```python
from build123d import *

# Parameters (mm, degrees)
CHAMFER_1_SIZE = 3


with BuildPart() as part:
    # Эскиз1 → Повернуть1 (revolve)
    with BuildSketch(Plane.XY):
        Polygon((9, 0), (20, 0), (20, 3.5), (15, 3.5), (15, 8), (12, 36), (5.5, 36), (5.5, 33), (9, 33), align=None)
    revolve(axis=Axis((0, 0, 0), (0, 1, 0)))

    # Эскиз2 → Вырез-Повернуть1 (revolve, cut)
    with BuildSketch(Plane.XY):
        with BuildLine():
            Line((13.5, -3.5), (13.5, -0.5))
            ThreePointArc((13.5, -0.5), (15.5, 1.5), (17.5, -0.5))
            Line((17.5, -0.5), (17.5, -3.5))
            ThreePointArc((17.5, -3.5), (15.5, -5.5), (13.5, -3.5))
        make_face()
    revolve(axis=Axis((0, 0, 0), (0, 1, 0)), mode=Mode.SUBTRACT)

    # Фаска1
    chamfer_1_edges = [part.edges().sort_by_distance(p)[0] for p in [
        (-9, 0, 0),
    ]]
    chamfer(chamfer_1_edges, length=CHAMFER_1_SIZE)


solid = part.part
```
Geometry: final body of the model. Coordinates: model frame, mm. A direction names the side the tool comes from. Coordinates: 2 decimals unless noted, no trailing zeros. Order: outer loops, then holes, each group sorted by start corner. A loop starts at its lowest first (then second) coordinate and runs counter-clockwise, first axis right, second up.
Item 1: Contact query for flat-ended pins moving along their axis: P1, Ø14.5, axis at x = 0, z = 0, coming from the +Y side; P2, Ø14.5, axis at x = 2.5, z = -2.5, coming from the -Y side; P3, Ø1.5, axis at x = -6, y = 6, coming from the -Z side; P4, Ø3, axis at x = 12.5, y = 17, coming from the +Z side. Output: stop coordinate, or through.
Answer:
P1: stops at y = 36
P2: stops at y = 1.21
P3: stops at z = -14.05
P4: stops at z = 8.74
Item 2: Section query B-B (x = 0). Output: boundary loops of the cut face in (y, z).
Answer:
outline: (0, -20) - (3.5, -20) - (3.5, -15) - (8, -15) - (36, -12) - (36, -5.5) - (33, -5.5) - (33, -9) - (3, -9) - (0, -12) - (0, -13.56) arc R2 cw to (0, -17.44) - close; (0, 12) - (3, 9) - (33, 9) - (33, 5.5) - (36, 5.5) - (36, 12) - (8, 15) - (3.5, 15) - (3.5, 20) - (0, 20) - (0, 17.44) arc R2 cw to (0, 13.56) - close
Item 3: Material intervals for line 1 along Y through (x, z) = (17, 9.5); line 2 along Z through (x, y) = (6, 14); line 3 along X through (y, z) = (22.5, 0), sorted ascending.
Answer:
line 1: y = 0 to 3.5
line 2: z = -13.04 to -6.71, 6.71 to 13.04
line 3: x = -13.45 to -9, 9 to 13.45
Item 4: Section query C-C (y = 19). Output: boundary loops of the cut face in (x, z).
Answer:
outline: circle Ø27.64 at (0, 0); hole circle Ø18 at (0, 0)
Item 5: Section query A-A (z = 0). Output: boundary loops of the cut face in (x, y).
Answer:
outline: (-20, 0) - (-17.44, 0) arc R2 cw to (-13.56, 0) - (-12, 0) - (-9, 3) - (-9, 33) - (-5.5, 33) - (-5.5, 36) - (-12, 36) - (-15, 8) - (-15, 3.5) - (-20, 3.5) - close; (5.5, 33) - (9, 33) - (9, 3) - (12, 0) - (13.56, 0) arc R2 cw to (17.44, 0) - (20, 0) - (20, 3.5) - (15, 3.5) - (15, 8) - (12, 36) - (5.5, 36) - close
Item 6: Draft query along X for faces 1 (the face through (-14.985, 5.781, -0.66)), 2 (the face through (-7.258, 2.854, 5.565)), 3 (the face through (-1.19, 34.48, 5.37)), 4 (the face through (-3, 0, 12)). Return one class per face: released by +X, released by -X, zero draft, split by the parting line, or undercut.
Answer:
face 1: split by the parting line
face 2: undercut
face 3: undercut
face 4: zero draft
Item 7: Access query for faces 5 (the face through (3, 3.5, -15)), 6 (the face through (-4.336, 1.774, 19.524)), 7 (the face through (-1.172, 17.79, -8.923)). Directions: +Z, -Z, +X, -X, +Y, -Y. A direction counts if a zero-diameter tool reaches every point of the face in a straight line with its end or side. Return the directions, or none.
Answer:
face 5: +Y
face 6: +Y, -Y
face 7: -Y
Item 8: Section query D-D (y = 29.5). Output: boundary loops of the cut face in (x, z).
Answer:
outline: circle Ø25.39 at (0, 0); hole circle Ø18 at (0, 0)
